Geometry check sheet. Reference: the model listing, model coordinates, mm. A direction names the side the tool comes from. Round coordinates to 2 decimals unless told otherwise and drop trailing zeros. Write each loop counter-clockwise with the first axis right and the second up, starting at its lowest first coordinate (ties: lowest second). Pieces come first, ordered by that corner, then holes. Notation, with made-up numbers: (-21, 83) -> (30, 83) arc R16 cw to (30, 114) -> close; hole circle Ø3 at (-17, 26). An arc over 180 degrees is marked (long way). Put each result on its own line as item: value. Start each with the question number.
from build123d import *

# Parameters (mm, degrees)
SKETCH1_W               = 6
SKETCH1_H               = 40
BOSS_EXTRUDE1_DEPTH     = 60
SKETCH2_W               = 3.2
SKETCH2_H               = 40
CUT_EXTRUDE2_DEPTH      = 20
SKETCH3_R               = 2
CUT_EXTRUDE3_DEPTH      = 1
CUT_EXTRUDE3_DEPTH_BACK = 41
SKETCH4_R               = 4.5
BOSS_EXTRUDE2_DEPTH     = 40
SKETCH6_R               = 2
CUT_EXTRUDE4_DEPTH      = 40
SKETCH7_W               = 20.491200394
SKETCH7_H               = 6.65
CUT_EXTRUDE5_DEPTH      = 2.5
CUT_EXTRUDE5_DEPTH_BACK = 8.5
SKETCH8_R               = 4.5
CUT_EXTRUDE6_DEPTH      = 20.4912
SKETCH9_W               = 1.395608407
SKETCH9_H               = 40
SKETCH9_W_2             = 1.404391593
BOSS_EXTRUDE3_DEPTH     = 15
SKETCH10_W              = 3.2
SKETCH10_H              = 40
BOSS_EXTRUDE4_DEPTH     = 15


with BuildPart() as part:
    # Sketch1 → Boss-Extrude1 (new body)
    with BuildSketch(Plane(origin=(0, 0, 0), x_dir=(1, 0, 0), z_dir=(0, 1, 0))):
        with Locations((-39.19123506, 9.482071713)):
            Rectangle(SKETCH1_W, SKETCH1_H)
    extrude(amount=BOSS_EXTRUDE1_DEPTH)

    # Sketch2 → Cut-Extrude2 (cut)
    with BuildSketch(Plane.XZ):
        with Locations((-39.195626653, -9.482071713)):
            Rectangle(SKETCH2_W, SKETCH2_H)
    extrude(amount=-CUT_EXTRUDE2_DEPTH, mode=Mode.SUBTRACT)

    # Sketch3 → Cut-Extrude3 (cut, two sides)
    with BuildSketch(Plane.XY.offset(10.517928287)) as cut_extrude3_sk:
        with Locations((-39.19123506, 57.687817086)):
            Circle(SKETCH3_R)
    extrude(amount=CUT_EXTRUDE3_DEPTH, mode=Mode.SUBTRACT)
    extrude(cut_extrude3_sk.sketch, amount=-CUT_EXTRUDE3_DEPTH_BACK, mode=Mode.SUBTRACT)

    # Sketch4 → Boss-Extrude2 (add)
    with BuildSketch(Plane.XY.offset(10.517928287)):
        with Locations((-39.19123506, 57.687817086)):
            Circle(SKETCH4_R)
    extrude(amount=-BOSS_EXTRUDE2_DEPTH)

    # Sketch6 → Cut-Extrude4 (cut)
    with BuildSketch(Plane.XY.offset(10.517928287)):
        with Locations((-39.19123506, 57.687817086)):
            Circle(SKETCH6_R)
    extrude(amount=-CUT_EXTRUDE4_DEPTH, mode=Mode.SUBTRACT)

    # Sketch7 → Cut-Extrude5 (cut, two sides)
    with BuildSketch(Plane(origin=(-36.19123506, 0, 0), x_dir=(0, 0, -1), z_dir=(1, 0, 0))) as cut_extrude5_sk:
        with Locations((9.482071713, 58.362817086)):
            Rectangle(SKETCH7_W, SKETCH7_H)
    extrude(amount=CUT_EXTRUDE5_DEPTH, mode=Mode.SUBTRACT)
    extrude(cut_extrude5_sk.sketch, amount=-CUT_EXTRUDE5_DEPTH_BACK, mode=Mode.SUBTRACT)

    # Sketch8 → Cut-Extrude6 (cut)
    with BuildSketch(Plane(origin=(0, 0, 0.763528484), x_dir=(-1, 0, 0), z_dir=(0, 0, -1))):
        with Locations((39.19123506, 57.687817086)):
            Circle(SKETCH8_R)
    extrude(amount=CUT_EXTRUDE6_DEPTH, mode=Mode.SUBTRACT)

    # Sketch9 → Boss-Extrude3 (add)
    with BuildSketch(Plane.XZ):
        with Locations((-41.493430856, -9.482071713)):
            Rectangle(SKETCH9_W, SKETCH9_H)
        with Locations((-36.893430857, -9.482071713)):
            Rectangle(SKETCH9_W_2, SKETCH9_H)
    extrude(amount=BOSS_EXTRUDE3_DEPTH)

    # Sketch10 → Boss-Extrude4 (add)
    with BuildSketch(Plane.XZ.offset(-20)):
        with Locations((-39.195626653, -9.482071713)):
            Rectangle(SKETCH10_W, SKETCH10_H)
    extrude(amount=BOSS_EXTRUDE4_DEPTH)


solid = part.part
(1) Set-up check for faces 1 (the flat face through (-36.191, 19, -9)), 2 (the flat face through (-42.191, 20, -10)), 3 (the cylindrical face through (-40.7, 59, 5.7)), 4 (the flat face through (-39, 5, -9)): record each of +Z, -Z, +X, -X, +Y, -Y from which the full face is reachable in a straight line by a thin tool's end or side.
(2) Sectioned sample at A-A (y = -3). Record the cut outline in (x, z).
(3) Sectioned sample at C-C (z = -8.5). Record the cut outline in (x, y), and give its area (3 significant figures).
(4) Mould release check, pull along Z, two halves, no side actions. Record for faces 5 (the cylindrical face through (-39.039, 62.185, -24.537)), 6 (the flat face through (-41.13, 56.75, 0.764)), 7 (the cylindrical face through (-39.15, 53.19, -9.34)), 8 (the flat face through (-38, 24, -29.482)): +Z half, -Z half, draft (parallel to the pull), parting line (faces both ways), or undercut.
(5) Go/stop test with flat-tipped pins: pin 1 Ø22 at (y, z) = (-5, -16.5) entering from -X; pin 2 Ø3 at (x, y) = (-39.19, 57.69) entering from +Z; pin 3 Ø5 at (x, y) = (-39.19, 57.69) entering from +Z; pin 4 Ø22 at (y, z) = (-8, -3.5) entering from +X. Record where each tip stops, or that it passes through.
(6) Sectioned sample at D-D (z = -25.5). Record the cut outline in (x, y), and give its area (3 significant figures).
(7) Material ranges on L1, parallel to Y at x = -39.25, z = -22.5; L2, parallel to X at y = -8, z = -3; L3, parallel to Z at x = -36.25, y = 59, recorded low to high. Write a range as from..to.
(8) Sectioned sample at B-B (x = -39.75). Record the cut outline in (y, z), and give its area (3 significant figures).
Found:
1. face 1: +Z, -Z, +X, -Y
1. face 2: +Z, -Z, -X, -Y
1. face 3: +Z, -Z
1. face 4: +Z, -Z, -Y
2. outline: (-42.19, -29.48) -> (-40.8, -29.48) -> (-40.8, 10.52) -> (-42.19, 10.52) -> close; (-37.6, -29.48) -> (-36.19, -29.48) -> (-36.19, 10.52) -> (-37.6, 10.52) -> close
3. outline: (-42.19, -15) -> (-40.8, -15) -> (-40.8, 5) -> (-37.6, 5) -> (-37.6, -15) -> (-36.19, -15) -> (-36.19, 54.33) arc R4.5 cw to (-42.19, 54.33) -> close
3. area: 347 mm2
4. face 5: draft
4. face 6: undercut
4. face 7: undercut
4. face 8: -Z half
5. pin 1: x = -42.19
5. pin 2: through
5. pin 3: z = 10.52
5. pin 4: x = -36.19
6. outline: (-42.19, -15) -> (-40.8, -15) -> (-40.8, 5) -> (-37.6, 5) -> (-37.6, -15) -> (-36.19, -15) -> (-36.19, 54.33) arc R4.5 ccw (long way) to (-42.19, 54.33) -> close; hole circle Ø4 at (-39.19, 57.69)
6. area: 398 mm2
7. L1: 5..55.69, 59.69..62.19
7. L2: -42.19..-40.8, -37.6..-36.19
7. L3: -29.48..-19.73, 0.76..10.52
8. outline: (5, -29.48) -> (55.77, -29.48) -> (55.77, -19.73) -> (53.22, -19.73) -> (53.22, 0.76) -> (55.77, 0.76) -> (55.77, 10.52) -> (5, 10.52) -> close; (59.61, -29.48) -> (62.15, -29.48) -> (62.15, -19.73) -> (59.61, -19.73) -> close; (59.61, 0.76) -> (62.15, 0.76) -> (62.15, 10.52) -> (59.61, 10.52) -> close
8. area: 2,030 mm2
